Geometry check sheet. Reference: the model listing, model coordinates, mm. Give positions to 0.01 mm unless a question says otherwise; leave off trailing zeros. Order: outer loops, then holes, each group sorted by start corner. A loop starts at its lowest first (then second) coordinate and runs counter-clockwise, first axis right, second up. Notation, with made-up numbers: M 43.25,1.5 L 91.25,1.5 A35 ccw 91.25,39.5 Z; hole C 42.25,-27.5 d11. An arc over 180 degrees is marked long. Answer as a JSON object with one key per item and string values. Group by question number.
Autodesk Inventor part; units mm, degrees
ref_plane "YZ Plane" through (0, 0, 0) normal (1, 0, 0) x (0, 1, 0)
ref_plane "XZ Plane" through (0, 0, 0) normal (0, 1, 0) x (-1, 0, 0)
ref_plane "XY Plane" through (0, 0, 0) normal (0, 0, 1) x (1, 0, 0)
sketch "Sketch1" plane through (0, 0, 0) normal (0, 0, 1) x (1, 0, 0)
  line L0 (150, 125) -> (110, 125)
  line L1 (110, 125) -> (110, -35)
  line L2 (110, -35) -> (150, -35)
  line L3 (150, -35) -> (150, 125)
  point P0 (0, 0)
  dimension "d0" = 40
  dimension "d3" = 160
extrude "Extrusion1" add sketch "Sketch1" along normal blind 5
ref_plane "Work Plane1" through (0, 0, 0) normal (0, 0, 1) x (1, 0, 0)
sketch "Sketch3" plane through (0, 0, 5) normal (0, 0, 1) x (1, 0, 0)
  line L0 (150, 125) -> (110, 125) construction
  line L1 (130, 125) -> (130, -35) construction
  line L2 (110, -35) -> (150, -35) construction
  line L3 (110, 125) -> (110, -35) construction
  line L4 (110, 45) -> (150, 45) construction
  line L5 (150, -35) -> (150, 125) construction
  point P0 (0, 0)
  point P1 (120, 115)
  point P2 (140, 115)
  point P3 (120, -25)
  point P4 (140, -25)
  dimension "d4" = 20
  dimension "d5" = 10
hole "Hole1" at (120, 115, 5) at (140, 115, 5) at (120, -25, 5) at (140, -25, 5) direction (0, 0, -1) diameter 5 end through all
properties part number "ReposadorPinzas" material "MDF Medium Density Fiberboard"
1. Depth check by flat-ended pin: pin 1 (5 mm diameter, centred on x = 123.5, y = 21, fed in from -Z); pin 2 (4 mm diameter, centred on x = 120, y = 115, fed in from +Z) (1 decimal). Enter the tip coordinate at first touch or a pass-through.
2. Cross-section at A-A (x = 120). Record the cut outline in (y, z).
3. Thickness scan on line 1 along Y through (x, z) = (120, 3.8); line 2 along X through (y, z) = (-25, 1.1); line 3 along Y through (x, z) = (122, 4.2). Record the ranges inside material, lowest first. Write a range as [from, to].
4. Cross-section at B-B (y = 115). Record the cut outline in (x, z).
5. Release check for a two-part mould opening along Y. For faces 1 (the cylindrical face through (117.52, -24.67, 2.46)), 2 (the cylindrical face through (137.52, -24.67, 2.46)), 3 (the flat face through (130, -35, 2)), 4 (the flat face through (130, 46, 0)) record: released by +Y, released by -Y, zero draft, split by the parting line, or undercut.
Report:
{
 "1": {"pin 1": "stops at z = 0", "pin 2": "passes through"},
 "2": {"outline": "M -35,0 L -27.5,0 L -27.5,5 L -35,5 Z; M -22.5,0 L 112.5,0 L 112.5,5 L -22.5,5 Z; M 117.5,0 L 125,0 L 125,5 L 117.5,5 Z"},
 "3": {"line 1": "y = [-35, -27.5], [-22.5, 112.5], [117.5, 125]", "line 2": "x = [110, 117.5], [122.5, 137.5], [142.5, 150]", "line 3": "y = [-35, -26.5], [-23.5, 113.5], [116.5, 125]"},
 "4": {"outline": "M 110,0 L 117.5,0 L 117.5,5 L 110,5 Z; M 122.5,0 L 137.5,0 L 137.5,5 L 122.5,5 Z; M 142.5,0 L 150,0 L 150,5 L 142.5,5 Z"},
 "5": {"face 1": "undercut", "face 2": "undercut", "face 3": "released by -Y", "face 4": "zero draft"}
}
